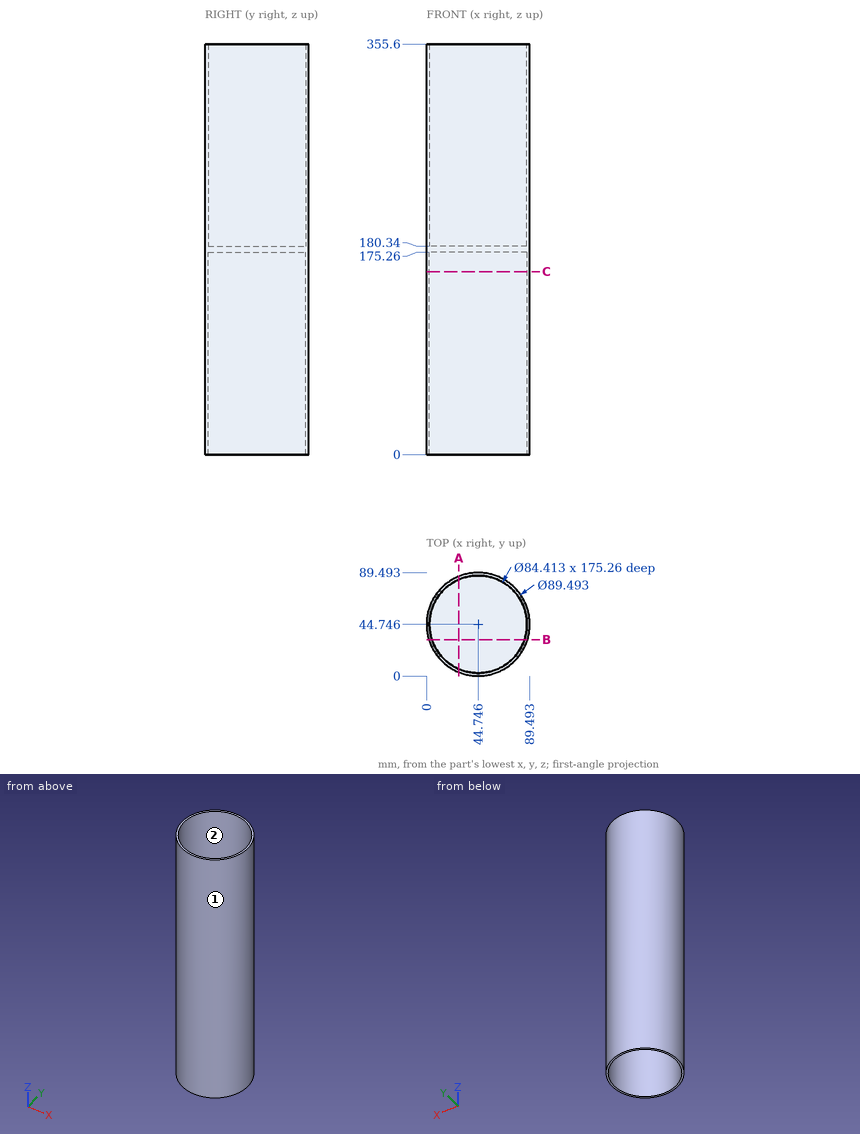
The figure shows three views and two pictorial views of one solid part (mm, origin at its lowest corner). Answer the questions. Coordinates: 2 decimals unless noted, no trailing zeros. Loops run counter-clockwise (first coordinate to the right, second up) from the corner with the lowest first, then second, coordinate; pieces in that order, holes last. Notation, with made-up numbers: (-5.5, -1.75) -> (36.5, -1.75) arc R16 ccw to (36.5, 21.25) -> close; hole circle Ø10 at (-39.75, -36.5). An arc over 180 degrees is marked (long way). Return JSON: item names as keys, results as strings. Group by question number.
(1) A cutting plane is placed at A-A on x = 28. Write down the section's boundary in (y, z) (1 decimal).
(2) Given pin 1 Ø2 at (y, z) = (60.5, 212) entering from -X; pin 2 Ø5 at (x, z) = (12, 258.5) entering from +Y; pin 3 Ø4 at (x, y) = (42.5, 33) entering from +Z, each flat-ended and moving along its own axis, determine where each tip first touches the part or whether it passes through.
(3) Find the intervals of material crossed by probe 1 along Z at (x, y) = (38.5, 63.5); probe 2 along X at (y, z) = (18, 168) (1 decimal); probe 3 along Y at (x, z) = (63.5, 198) (1 decimal), in increasing order. Write a range as from..to.
(4) A cutting plane is placed at C-C on z = 158.5. Write down the section's boundary in (x, y).
(5) Determine the mould class of the marked faces 1 and 2 for opening direction X: released by +X, released by -X, zero draft, split by the parting line, or undercut.
(6) A cutting plane is placed at B-B on y = 31.5. Write down the section's boundary in (x, z) (1 decimal).
The answers:
{
 "1": {"outline": "(3.3, 0) -> (6, 0) -> (6, 175.3) -> (83.5, 175.3) -> (83.5, 0) -> (86.2, 0) -> (86.2, 355.6) -> (83.5, 355.6) -> (83.5, 180.3) -> (6, 180.3) -> (6, 355.6) -> (3.3, 355.6) -> close"},
 "2": {"pin 1": "stops at x = 2.5", "pin 2": "stops at y = 77.72", "pin 3": "stops at z = 180.34"},
 "3": {"probe 1": "z = 175.26..180.34", "probe 2": "x = 8.9..12.1, 77.4..80.6", "probe 3": "y = 4.1..6.9, 82.6..85.4"},
 "4": {"outline": "circle Ø89.49 at (44.75, 44.75); hole circle Ø84.41 at (44.75, 44.75)"},
 "5": {"face 1": "split by the parting line", "face 2": "undercut"},
 "6": {"outline": "(2, 0) -> (4.7, 0) -> (4.7, 175.3) -> (84.8, 175.3) -> (84.8, 0) -> (87.5, 0) -> (87.5, 355.6) -> (84.8, 355.6) -> (84.8, 180.3) -> (4.7, 180.3) -> (4.7, 355.6) -> (2, 355.6) -> close"}
}
